The listing builds one solid part. Answer for the finished solid, in the listing's coordinates (mm). Face numbers are marked on the shaded views. A direction names the side the tool comes from. Give positions to 0.01 mm unless a question says otherwise; leave off trailing zeros. Write each loop counter-clockwise with the first axis right and the second up, starting at its lowest first coordinate (ties: lowest second). Pieces come first, ordered by that corner, then holes.
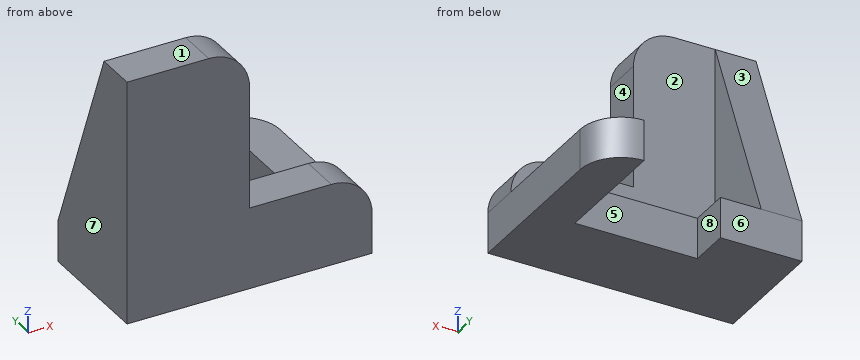
Autodesk Inventor part; units mm, degrees
ref_plane "YZ Plane" through (0, 0, 0) normal (1, 0, 0) x (0, 1, 0)
ref_plane "XZ Plane" through (0, 0, 0) normal (0, 1, 0) x (-1, 0, 0)
ref_plane "XY Plane" through (0, 0, 0) normal (0, 0, 1) x (1, 0, 0)
sketch "草圖1" plane through (0, 0, 0) normal (0, 1, 0) x (-1, 0, 0)
  line L0 (0, 0) -> (0, 60)
  line L1 (-60, 10) -> (-60, 0)
  line L2 (-60, 0) -> (0, 0)
  line L3 (0, 60) -> (-20, 60)
  arc A0 (-20, 60) -> (-30, 50) centre (-20, 50) ccw
  line L4 (-30, 50) -> (-30, 20)
  line L5 (-30, 20) -> (-50, 20)
  arc A1 (-50, 20) -> (-60, 10) centre (-50, 10) ccw
  dimension "d0" = 60
  dimension "d1" = 10
  dimension "d2" = 20
  dimension "d3" = 60
  dimension "d4" = 30
  dimension "d5" = 20
extrude "擠出1" add sketch "草圖1" along normal blind 10
sketch "草圖2" plane through (60, 0, 0) normal (0, 0, -1) x (-1, 0, 0)
  line L0 (0, 0) -> (0, 10)
  line L1 (0, 10) -> (60, 10)
  line L2 (60, 10) -> (60, 0)
  line L3 (60, 0) -> (0, 0)
  line L4 (0, 10) -> (0, 40)
  arc A0 (10, 50) -> (0, 40) centre (10, 40) ccw
  line L5 (10, 50) -> (10, 20)
  line L6 (10, 20) -> (40, 20)
  line L7 (40, 20) -> (40, 30)
  line L8 (40, 30) -> (60, 30)
  line L9 (60, 30) -> (60, 10)
  dimension "d8" = 30
  dimension "d9" = 20
  dimension "d10" = 10
  dimension "d11" = 20
  dimension "d12" = 50
extrude "擠出2" add sketch "草圖2" against normal blind 10 contours L4 A0 L5 L6 L7 L8 L9 L1
sketch "草圖3" plane through (0, 0, 0) normal (-1, 0, 0) x (0, 0, 1)
  line L0 (0, 30) -> (10, 30)
  line L1 (10, 30) -> (10, 10)
  line L2 (10, 10) -> (60, 10)
  line L3 (60, 10) -> (60, 0)
  line L4 (60, 0) -> (0, 0)
  line L5 (0, 0) -> (0, 30)
  line L6 (60, 10) -> (10, 30)
extrude "擠出3" add sketch "草圖3" against normal blind 10 contours L6 L2 L1
properties part number "5" material "鋼、碳鋼"
Item 1: A cutting plane is placed at A-A, the plane y = 23.5. Give the vertices of the cut face in (x, z), plus the area to 4 significant figures.
Conclusion:
outline: (0, 0) - (20, 0) - (20, 10) - (10, 10) - (10, 26.25) - (0, 26.25) - close; (50, 0) - (60, 0) - (60, 10) - (50, 10) - close
area: 462.5 mm2
Item 2: Each of these flat-tipped pins is pushed along its axis until it touches: P1, Ø3, axis at x = 19.5, z = 29, coming from the +Y side; P2, Ø5, axis at y = 7.5, z = 38, coming from the +X side; P3, Ø5, axis at x = 9.5, z = 7, coming from the +Y side. Where does it stop, or does it pass through?
Conclusion:
P1: stops at y = 10
P2: stops at x = 30
P3: stops at y = 30
Item 3: Which of the six approach directions +Z, -Z, +X, -X, +Y, -Y give full straight-line access (tool end or side, diameter ignored) to the marked faces 1, 2, 3, 4 and 5?
Conclusion:
face 1: +Z, +X, -X, +Y, -Y
face 2: +Z, +X, +Y
face 3: +Z, +X, -X, +Y
face 4: +Z, +X, +Y, -Y
face 5: +Z, -Z, +Y
Item 4: Consider probe 1 along Z at (x, y) = (36.5, 11); probe 2 along Z at (x, y) = (36, 3). Determine where each line is inside the solid, lowest interval first.
Conclusion:
probe 1: z = 0 to 10
probe 2: z = 0 to 20
Item 5: A cutting plane is placed at D-D, the plane x = 7. Give the vertices of the cut face in (y, z), plus the area to 3 significant figures.
Conclusion:
outline: (0, 0) - (30, 0) - (30, 10) - (10, 60) - (0, 60) - close
area: 1,300 mm2
Item 6: A cutting plane is placed at B-B, the plane z = 32. Give the vertices of the cut face in (x, y), plus the area to 3 significant figures.
Conclusion:
outline: (0, 0) - (30, 0) - (30, 10) - (10, 10) - (10, 21.2) - (0, 21.2) - close
area: 412 mm2
Item 7: Determine the mould class of the marked faces 6, 7 and 8 for opening direction X: pulls with the +X half, pulls with the -X half, needs draft (parallel to the pull), parting line crosses it, or undercut.
Conclusion:
face 6: needs draft
face 7: pulls with the -X half
face 8: undercut
Item 8: A cutting plane is placed at C-C, the plane y = 17. Give the vertices of the cut face in (x, z), plus the area to 3 significant figures.
Conclusion:
outline: (0, 0) - (60, 0) - (60, 10) - (10, 10) - (10, 42.5) - (0, 42.5) - close
area: 925 mm2
